from build123d import *

# Parameters (mm, degrees)
F0_R     = 279.4
F1_DEPTH = 736.6
F2_W     = 195.749157
F2_H     = 25.4
F2_W_2   = 25.4
F2_H_2   = 195.749157
F3_DEPTH = 1010.92


with BuildPart() as f1:
    # F0 (on Top) → F1 (new body)
    with BuildSketch(Plane.XY):
        Circle(F0_R)
    extrude(amount=F1_DEPTH)

    # F2 (on Top) → F3 (cut)
    with BuildSketch(Plane.XY):
        with Locations((0.382937, 277.498556)):
            Rectangle(F2_W, F2_H)
        with Locations((-277.498556, 0.382937)):
            Rectangle(F2_W_2, F2_H_2)
        with Locations((-0.382937, -277.498556)):
            Rectangle(F2_W, F2_H)
        with Locations((277.498556, -0.382937)):
            Rectangle(F2_W_2, F2_H_2)
    extrude(amount=F3_DEPTH, mode=Mode.SUBTRACT)


solid = f1.part
Verification items for the finished model (mm, model axes). Give positions to 0.01 mm unless a question says otherwise; leave off trailing zeros. Write each loop counter-clockwise with the first axis right and the second up, starting at its lowest first coordinate (ties: lowest second). Pieces come first, ordered by that corner, then holes. Notation, with made-up numbers: M -4.5,10 L 47.5,10 A20 ccw 47.5,43 Z; hole C 74.25,34.25 d2. An arc over 180 degrees is marked long. Use CSV: the item, a comma, the result in double quotes.
1) Go/stop test with flat-tipped pins: pin 1 Ø12 at (y, z) = (-136, 381.5) entering from -X; pin 2 Ø5 at (x, z) = (104, 298.5) entering from -Y; pin 3 Ø5 at (x, z) = (-116, 131) entering from +Y. Record where each tip stops, or that it passes through.
Final values:
pin 1,"x = -247.31"
pin 2,"y = -260.31"
pin 3,"y = 255.31"
2) Cross-section at B-B (y = -175). Enter the section's corners in (x, z), plus the area to 3 significant figures.
Final values:
outline,"M -217.81,0 L 217.81,0 L 217.81,736.6 L -217.81,736.6 Z"
area,"321,000 mm²"
3) Cross-section at C-C (x = -156). Enter the section's corners in (y, z), plus the area to 3 significant figures.
Final values:
outline,"M -231.79,0 L 231.79,0 L 231.79,736.6 L -231.79,736.6 Z"
area,"341,000 mm²"
4) Material ranges on line 1 along Y through (x, z) = (139, 690); line 2 along X through (y, z) = (-233.5, 306); line 3 along Y through (x, z) = (152.5, 159.5), recorded low to high.
Final values:
line 1,"-242.37 to 242.37"
line 2,"-153.43 to 153.43"
line 3,"-234.11 to 234.11"
5) Cross-section at A-A (z = 330). Enter the section's corners in (x, y), plus the area to 3 significant figures.
Final values:
outline,"M -264.8,-89.14 A279.4 ccw -89.14,-264.8 L 89.14,-264.8 A279.4 ccw 264.8,-89.14 L 264.8,89.14 A279.4 ccw 89.14,264.8 L -89.14,264.8 A279.4 ccw -264.8,89.14 Z"
area,"238,000 mm²"
